Geometry: final body of the model. Coordinates: model frame, mm. Give positions to 0.01 mm unless a question says otherwise; leave off trailing zeros. Loops run counter-clockwise (first coordinate to the right, second up) from the corner with the lowest first, then second, coordinate; pieces in that order, holes last. Notation, with made-up numbers: (83, 23.5) - (87, 23.5) arc R18 ccw to (87, 36.5) - close; hole circle Ø6 at (-30.5, 80.5). An arc over 180 degrees is marked (long way). Use one line per item in the form item = value.
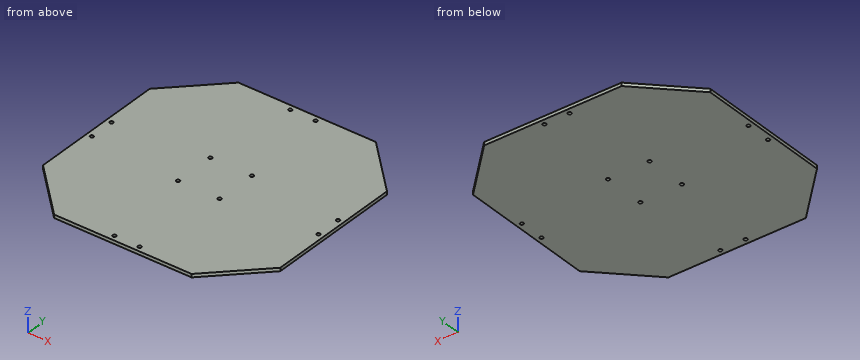
```python
from build123d import *

# Parameters (mm, degrees)
BOSS_EXTRUDE1_DEPTH  = 3.175
M3_CLEARANCE_HOLE1_D = 3.4
SKETCH6_R            = 1.651
CUT_EXTRUDE1_DEPTH   = 3.175


with BuildPart() as part:
    # Sketch1 → Boss-Extrude1 (new body)
    with BuildSketch(Plane.XY):
        Polygon((-88.939961868, 77.031330301), (-40.856700747, 28.948069181), (91.576777011, 28.948069181), (139.660038132, 77.031330301), (139.660038132, 209.46480806), (91.576777011, 257.548069181), (-40.856700747, 257.548069181), (-88.939961868, 209.46480806), align=None)
    extrude(amount=BOSS_EXTRUDE1_DEPTH)

    # M3 Clearance Hole1 (through all)
    with Locations(Plane.XY.offset(3.175)):
        with Locations((5.360038132, 163.248069181), (45.360038132, 123.248069181), (45.360038132, 163.248069181), (5.360038132, 123.248069181)):
            Hole(M3_CLEARANCE_HOLE1_D / 2)

    # Sketch6 → Cut-Extrude1 (cut)
    with BuildSketch(Plane.XY.offset(3.175)):
        with Locations((37.560038132, 252.391869181)):
            Circle(SKETCH6_R)
        with Locations((13.160038132, 252.391869181)):
            Circle(SKETCH6_R)
        with Locations((-83.783761868, 155.448069181)):
            Circle(SKETCH6_R)
        with Locations((-83.783761868, 131.048069181)):
            Circle(SKETCH6_R)
        with Locations((13.160038132, 34.104269181)):
            Circle(SKETCH6_R)
        with Locations((37.560038132, 34.104269181)):
            Circle(SKETCH6_R)
        with Locations((134.503838132, 131.048069181)):
            Circle(SKETCH6_R)
        with Locations((134.503838132, 155.448069181)):
            Circle(SKETCH6_R)
    extrude(amount=-CUT_EXTRUDE1_DEPTH, mode=Mode.SUBTRACT)


solid = part.part
```
(1) Cut plane C-C (x = 117.5). Return the cut outline in (y, z) (3 decimals).
Solution:
outline = (54.871, 0) - (231.625, 0) - (231.625, 3.175) - (54.871, 3.175) - close
(2) Cut plane A-A (z = 2.2). Give the number of separate pieces and of enclosed holes in the cut face, plus the area to 3 significant figures.
Solution:
separate_pieces = 1
enclosed_holes = 12
area = 47,500 mm2
(3) Material intervals for L1, parallel to Y at x = -74, z = 1.25; L2, parallel to X at y = 238, z = 0.5; L3, parallel to Y at x = 92.5, z = 0.9, sorted ascending. Write a range as from..to.
Solution:
L1 = 62.09..224.4
L2 = -60.4..111.12
L3 = 29.87..256.62
(4) Cut plane B-B (y = 219). Return the cut outline in (x, z) (3 decimals).
Solution:
outline = (-79.405, 0) - (130.125, 0) - (130.125, 3.175) - (-79.405, 3.175) - close
(5) Pin query (flat end, axial travel): P1, Ø2, axis at x = 13.16, y = 34.1, coming from the -Z side. Return the tip coordinate at first contact, or that it passes through.
Solution:
P1 = through
